from build123d import *

# Parameters (mm, degrees)
F0_R     = 8.5725
F1_DEPTH = 3.175
F2_R     = 19.05
F3_R     = 4.7625


with BuildPart() as f1:
    # F0 (on Top) → F1 (new body)
    with BuildSketch(Plane.XY):
        Polygon((-22.126334, 214.595574), (-130.076334, 214.595574), (-130.076334, -220.379426), (-22.126334, -220.379426), (-22.126334, -169.579426), (-31.651334, -169.579426), (-31.651334, 132.045574), (-22.126334, 132.045574), align=None)
        with Locations((-102.999538, -193.391926)):
            Circle(F0_R, mode=Mode.SUBTRACT)
        with Locations((-102.999538, 187.608074)):
            Circle(F0_R, mode=Mode.SUBTRACT)
    extrude(amount=F1_DEPTH)

    # F2
    f2_edges = [f1.edges().sort_by_distance(p)[0] for p in [
        (-130.076334, -220.379426, 1.5875),
        (-22.126334, -220.379426, 1.5875),
        (-130.076334, 214.595574, 1.5875),
        (-22.126334, 214.595574, 1.5875),
    ]]
    fillet(f2_edges, radius=F2_R)

    # F3
    f3_edges = [f1.edges().sort_by_distance(p)[0] for p in [
        (-31.651334, -169.579426, 1.5875),
        (-31.651334, 132.045574, 1.5875),
    ]]
    fillet(f3_edges, radius=F3_R)


solid = f1.part
Verification items for the finished model (mm, model axes). Round coordinates to 2 decimals unless told otherwise and drop trailing zeros. Order: outer loops, then holes, each group sorted by start corner. A loop starts at its lowest first (then second) coordinate and runs counter-clockwise, first axis right, second up.
1. Section check C-C on x = -122. Record the cut outline in (y, z) (3 decimals), then the cut area to 3 significant figures.
Final values:
outline: (-216.901, 0) - (211.117, 0) - (211.117, 3.175) - (-216.901, 3.175) - close
area: 1,360 mm2
2. Section check B-B on y = -68. Record the cut outline in (x, z) (3 decimals).
Final values:
outline: (-130.076, 0) - (-31.651, 0) - (-31.651, 3.175) - (-130.076, 3.175) - close
3. Release check for a two-part mould opening along X. For faces 1 (the flat face through (-77, 0, 3.175)), 2 (the cylindrical face through (-104.86, 179.24, 1.57)), 3 (the cylindrical face through (-124.35, 209.16, 1.61)), 4 (the cylindrical face through (-27.855, -214.947, 1.61)) record: +X half, -X half, draft (parallel to the pull), parting line (faces both ways), or undercut.
Final values:
face 1: draft
face 2: undercut
face 3: -X half
face 4: +X half
4. Thickness scan on L1, parallel to X at y = -144.5, z = 2.9; L2, parallel to X at y = 187.5, z = 2.15; L3, parallel to X at y = 191, z = 0.85. Record the ranges inside material, lowest first.
Final values:
L1: x = -130.08 to -31.65
L2: x = -130.08 to -111.57, -94.43 to -22.13
L3: x = -130.08 to -110.87, -95.13 to -22.13
5. Section check A-A on z = 0.5. State how many separate pieces and enclosed holes the cut face has, then the cut area to 3 significant figures.
Final values:
separate pieces: 1
enclosed holes: 2
area: 43,300 mm2
6. Go/stop test with a flat-tipped pin: P1, Ø13.5, axis at x = -103, y = -193.39, coming from the -Z side. Record where the tip stops, or that it passes through.
Final values:
P1: passes through
